Here's how the part is built. I have some questions about the finished solid (model axes, mm). A direction names the side the tool comes from. Coordinates: 2 decimals unless noted, no trailing zeros. Write each loop counter-clockwise with the first axis right and the second up, starting at its lowest first coordinate (ties: lowest second). Pieces come first, ordered by that corner, then holes. Notation, with made-up numbers: (47, -0.5) -> (78, -0.5) arc R27 cw to (78, 22.5) -> close; hole circle Ø1 at (89.5, -5). An arc over 180 degrees is marked (long way). Answer in a Markdown table with one row per item. Add a question column.
from build123d import *

# Parameters (mm, degrees)
F0_W     = 85
F0_H     = 15
F0_R     = 2.25
F0_R_2   = 1.75
F1_DEPTH = 2
F2_R     = 1.5
F3_R     = 3


# Not quite as in the source:
# - a feature names something its author has since deleted; it is built from what else it names


with BuildPart() as f1:
    # F0 (on Front) → F1 (new body)
    with BuildSketch(Plane.XZ):
        with Locations((0, 22.5)):
            Rectangle(F0_W, F0_H)
        with Locations((-37.5, 25)):
            Circle(F0_R, mode=Mode.SUBTRACT)
        with Locations((37.5, 25)):
            Circle(F0_R, mode=Mode.SUBTRACT)
        with Locations((0, -22.5)):
            Rectangle(F0_W, F0_H)
        with Locations((-37.5, -25)):
            Circle(F0_R, mode=Mode.SUBTRACT)
        with Locations((37.5, -25)):
            Circle(F0_R, mode=Mode.SUBTRACT)
        with BuildLine():
            Line((-42.5, -2), (-42.5, -15))
            Line((-42.5, -15), (42.5, -15))
            Line((42.5, -15), (42.5, -2))
            ThreePointArc((42.5, -2), (40.5, 0), (42.5, 2))
            Line((42.5, 2), (42.5, 15))
            Line((42.5, 15), (-42.5, 15))
            Line((-42.5, 15), (-42.5, 2))
            ThreePointArc((-42.5, 2), (-40.5, 0), (-42.5, -2))
        make_face()
        Circle(F0_R_2, mode=Mode.SUBTRACT)
        with BuildLine():
            Line((-65, -15), (-42.5, -15))
            Line((-42.5, -15), (-42.5, -2))
            Line((-42.5, -2), (-48, -2))
            Line((-48, -2), (-48, -7.5))
            ThreePointArc((-48, -7.5), (-50, -9.5), (-52, -7.5))
            Line((-52, -7.5), (-52, -2))
            Line((-52, -2), (-57.5, -2))
            ThreePointArc((-57.5, -2), (-59.5, 0), (-57.5, 2))
            Line((-57.5, 2), (-52, 2))
            Line((-52, 2), (-52, 7.5))
            ThreePointArc((-52, 7.5), (-50, 9.5), (-48, 7.5))
            Line((-48, 7.5), (-48, 2))
            Line((-48, 2), (-42.5, 2))
            Line((-42.5, 2), (-42.5, 15))
            Line((-42.5, 15), (-65, 15))
            Line((-65, 15), (-65, -15))
        make_face()
        with BuildLine():
            Line((42.5, -2), (42.5, -15))
            Line((42.5, -15), (65, -15))
            Line((65, -15), (65, 15))
            Line((65, 15), (42.5, 15))
            Line((42.5, 15), (42.5, 2))
            Line((42.5, 2), (48, 2))
            Line((48, 2), (48, 7.5))
            ThreePointArc((48, 7.5), (50, 9.5), (52, 7.5))
            Line((52, 7.5), (52, 2))
            Line((52, 2), (57.5, 2))
            ThreePointArc((57.5, 2), (59.5, 0), (57.5, -2))
            Line((57.5, -2), (52, -2))
            Line((52, -2), (52, -7.5))
            ThreePointArc((52, -7.5), (50, -9.5), (48, -7.5))
            Line((48, -7.5), (48, -2))
            Line((48, -2), (42.5, -2))
        make_face()
    extrude(amount=-F1_DEPTH)

    # F2
    f2_edges = [f1.edges().sort_by_distance(p)[0] for p in [
        (-42.5, 1, 30),
        (42.5, 1, 30),
        (42.5, 1, -30),
        (-42.5, 1, -30),
        (-42.5, 1, 15),
        (-65, 1, 15),
        (-65, 1, -15),
        (-42.5, 1, -15),
        (42.5, 1, 15),
        (65, 1, 15),
        (42.5, 1, -15),
        (65, 1, -15),
    ]]
    fillet(f2_edges, radius=F2_R)

    # F3
    f3_edges = [f1.edges().sort_by_distance(p)[0] for p in [
        (48, 1, 2),
        (52, 1, 2),
        (48, 1, -2),
        (52, 1, -2),
        (-48, 1, 2),
        (-52, 1, 2),
        (-48, 1, -2),
        (-52, 1, -2),
    ]]
    fillet(f3_edges, radius=F3_R)


solid = f1.part
Q1. Imagine slicing it at D-D on z = 25. Please give me the cut outline in (x, y).
Q2. I'm going to push flat-ended pins straight in: P1, Ø1, axis at x = 43.5, y = 1.5, coming from the +Z side; P2, Ø0.6, axis at x = 44, y = 1, coming from the -Z side; P3, Ø0.6, axis at y = 1.5, z = 24, coming from the +X side. Where does each tip first touch, or does it pass through?
Q3. Imagine slicing it at A-A on x = 0. Please give me the cut outline in (y, z), plus the area to 3 significant figures.
Q4. If we mould it in two halves opening along X, with no side actions, what happens to faces 3 (the cylindrical face through (47.14, 1.01, -2.9)), 4 (the flat face through (-1, 2, 7))? For each: pulls with the +X half, pulls with the -X half, needs draft (parallel to the pull), parting line crosses it, or undercut.
Q5. For faces 1 (the cylindrical face through (-52.86, 1.01, -2.9)), 2 (the flat face through (-1, 0, 7)), which set-ups out of +Z, -Z, +X, -X, +Y, -Y let a thin tool reach every point of the face, with its end or its side?
Q6. I need wall thicknesses on line 1 (Z direction, x = 37.5, y = 0.8); line 2 (X direction, y = 0.8, z = -8); line 3 (X direction, y = 0.95, z = -23.5). Which ranges of each line are inside material? Lowest first, please. Write a range as [from, to].
Q7. Imagine slicing it at B-B on z = 0. Please give me the cut outline in (x, y).
Q8. Imagine slicing it at C-C on x = -37.5. Please give me the cut outline in (y, z), plus the area to 3 significant figures.
Result sheet:
| question | item | result |
|---|---|---|
| 1 | outline | (-42.5, 0) -> (-39.75, 0) -> (-39.75, 2) -> (-42.5, 2) -> close; (-35.25, 0) -> (35.25, 0) -> (35.25, 2) -> (-35.25, 2) -> close; (39.75, 0) -> (42.5, 0) -> (42.5, 2) -> (39.75, 2) -> close |
| 2 | P1 | stops at z = 15.38 |
| 2 | P2 | stops at z = -15.03 |
| 2 | P3 | stops at x = 42.5 |
| 3 | outline | (0, -30) -> (2, -30) -> (2, -1.75) -> (0, -1.75) -> close; (0, 1.75) -> (2, 1.75) -> (2, 30) -> (0, 30) -> close |
| 3 | area | 113 mm^2 |
| 4 | face 3 | undercut |
| 4 | face 4 | needs draft |
| 5 | face 1 | +Y, -Y |
| 5 | face 2 | +Z, -Z, +X, -X, -Y |
| 6 | line 1 | z = [-30, -27.25], [-22.75, 22.75], [27.25, 30] |
| 6 | line 2 | x = [-65, -51.94], [-48.06, 48.06], [51.94, 65] |
| 6 | line 3 | x = [-42.5, -39.18], [-35.82, 35.82], [39.18, 42.5] |
| 7 | outline | (-65, 0) -> (-59.5, 0) -> (-59.5, 2) -> (-65, 2) -> close; (-40.5, 0) -> (-1.75, 0) -> (-1.75, 2) -> (-40.5, 2) -> close; (1.75, 0) -> (40.5, 0) -> (40.5, 2) -> (1.75, 2) -> close; (59.5, 0) -> (65, 0) -> (65, 2) -> (59.5, 2) -> close |
| 8 | outline | (0, -30) -> (2, -30) -> (2, -27.25) -> (0, -27.25) -> close; (0, -22.75) -> (2, -22.75) -> (2, 22.75) -> (0, 22.75) -> close; (0, 27.25) -> (2, 27.25) -> (2, 30) -> (0, 30) -> close |
| 8 | area | 102 mm^2 |
